Autodesk Inventor part; units mm, degrees
ref_plane "Work Plane7" through (0, 0, 15) normal (0, 0, 1) x (1, 0, 0)
ref_plane "Work Plane4" through (0, 0, 28) normal (0, 0, 1) x (1, 0, 0)
ref_plane "YZ Plane" through (0, 0, 0) normal (1, 0, 0) x (0, 1, 0)
ref_plane "Work Plane7" through (0, 0, 15) normal (0, 0, 1) x (1, 0, 0)
sketch "Sketch6" plane through (0, 0, 15) normal (0, 0, 1) x (1, 0, 0)
  circle A0 centre (0, 0) radius 1.7038
  dimension "d21" = 3.4076
extrude "Extrusion2" add sketch "Sketch6" along normal blind 10
ref_plane "Work Plane4" through (0, 0, 28) normal (0, 0, 1) x (1, 0, 0)
sketch "Sketch7" plane through (0, 0, 28) normal (0, 0, 1) x (1, 0, 0)
  arc A0 (-0.635, 0.635) -> (-0.635, -0.635) centre (-0.635, 0) ccw
  arc A1 (0.635, -0.635) -> (0.635, 0.635) centre (0.635, 0) ccw
  line L0 (-0.635, 0.635) -> (0.635, 0.635)
  line L1 (0.635, -0.635) -> (-0.635, -0.635)
loft "Loft4" add profiles "Sketch7" section 1 edges at (-1.7038, 0, 25)
sketch "Sketch8" plane through (0, 0, 28) normal (0, 0, 1) x (1, 0, 0)
  arc A0 (-0.635, 0.635) -> (-0.635, -0.635) centre (-0.635, 0) ccw
  circle A1 centre (-0.635, 0) radius 0.635
  arc A2 (0.635, -0.635) -> (0.635, 0.635) centre (0.635, 0) ccw
  circle A3 centre (0.635, 0) radius 0.635
  point P0 (0, 0)
extrude "Extrusion3" add sketch "Sketch8" along normal blind 25.4
sketch "Sketch9" plane through (0, 0, 15) normal (0, 0, -1) x (-1, 0, 0)
  circle A0 centre (0, 0) radius 1.25
  dimension "d36" = 2.5
extrude "Extrusion4" add sketch "Sketch9" along normal blind 15.0114
properties part number "Male End Audio Jack"
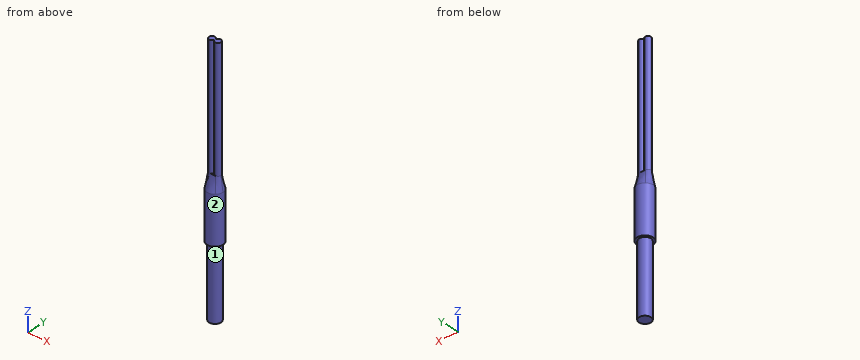
Geometry: final body of the model. Coordinates: model frame, mm. Face numbers are marked on the shaded views. A direction names the side the tool comes from. Round coordinates to 2 decimals unless told otherwise and drop trailing zeros. Order: outer loops, then holes, each group sorted by start corner. A loop starts at its lowest first (then second) coordinate and runs counter-clockwise, first axis right, second up. Notation, with made-up numbers: M 33.25,81.25 L 64.25,81.25 A24 ccw 64.25,110.25 Z; hole C -15.5,12.25 d10. An arc over 180 degrees is marked long. One line per item, written item: value.
(1) Cut plane B-B (z = 24). Return the cut outline in (x, y).
Result sheet:
outline: C 0,0 d3.41
(2) Pin query (flat end, axial travel): P1, Ø1.5, axis at x = -0.5, z = 36.5, coming from the -Y side (3 decimals). Return the tip coordinate at first contact, or that it passes through.
Result sheet:
P1: y = -0.635
(3) Line query: probe 1 along X at (y, z) = (0.3, 13); probe 2 along Y at (x, z) = (0.7, 38.5); probe 3 along X at (y, z) = (0.4, 30). Output: solid intervals per line, ascending. Write a range as [from, to].
Result sheet:
probe 1: [-1.21, 1.21]
probe 2: [-0.63, 0.63]
probe 3: [-1.13, -0.14], [0.14, 1.13]
(4) Reachability of the marked faces 1 and 2 from +Z, -Z, +X, -X, +Y, -Y: full face, straight path, thin tool, end or side. Return the list, or none.
Result sheet:
face 1: -Z
face 2: +Z, -Z
(5) Cut plane C-C (z = 12). Return the cut outline in (x, y), and give its area (3 significant figures).
Result sheet:
outline: C 0,0 d2.5
area: 4.91 mm2
